```python
from build123d import *

# Parameters (mm, degrees)
SKETCH1_R           = 41.275
SKETCH1_R_2         = 6.5024
SKETCH1_R_3         = 7.62
BOSS_EXTRUDE1_DEPTH = 9.525
SKETCH2_R           = 38.0365
SKETCH2_R_2         = 33.02
BOSS_EXTRUDE2_DEPTH = 63.5
SKETCH3_R           = 12.7
SKETCH3_R_2         = 6.5024
BOSS_EXTRUDE3_DEPTH = 15.875
CHAMFER1_SIZE       = 6.35
CHAMFER1_SIZE2      = 2.54
SKETCH4_R           = 12.7
SKETCH4_R_2         = 6.5024
BOSS_EXTRUDE4_DEPTH = 6.35
FILLET1_R           = 2.54


with BuildPart() as part:
    # Sketch1 → Boss-Extrude1 (new body)
    with BuildSketch(Plane(origin=(0, 0, 0), x_dir=(1, 0, 0), z_dir=(0, 1, 0))):
        Circle(SKETCH1_R)
        Circle(SKETCH1_R_2, mode=Mode.SUBTRACT)
        with Locations((0, 22.86)):
            Circle(SKETCH1_R_3, mode=Mode.SUBTRACT)
        with Locations((21.741151963, 7.064128491)):
            Circle(SKETCH1_R_3, mode=Mode.SUBTRACT)
        with Locations((13.436770867, -18.494128491)):
            Circle(SKETCH1_R_3, mode=Mode.SUBTRACT)
        with Locations((-13.436770867, -18.494128491)):
            Circle(SKETCH1_R_3, mode=Mode.SUBTRACT)
        with Locations((-21.741151963, 7.064128491)):
            Circle(SKETCH1_R_3, mode=Mode.SUBTRACT)
    extrude(amount=BOSS_EXTRUDE1_DEPTH)

    # Sketch2 → Boss-Extrude2 (add)
    with BuildSketch(Plane(origin=(0, 9.525, 0), x_dir=(1, 0, 0), z_dir=(0, 1, 0))):
        Circle(SKETCH2_R)
        Circle(SKETCH2_R_2, mode=Mode.SUBTRACT)
    extrude(amount=BOSS_EXTRUDE2_DEPTH)

    # Sketch3 → Boss-Extrude3 (add)
    with BuildSketch(Plane(origin=(0, 9.525, 0), x_dir=(1, 0, 0), z_dir=(0, 1, 0))):
        Circle(SKETCH3_R)
        Circle(SKETCH3_R_2, mode=Mode.SUBTRACT)
    extrude(amount=BOSS_EXTRUDE3_DEPTH)

    # Chamfer1
    chamfer1_edges = [part.edges().sort_by_distance(p)[0] for p in [
        (-38.0365, 73.025, 0),
    ]]
    chamfer1_side = [part.faces().sort_by_distance(p)[0] for p in [
        (-38.0365, 41.275, 0),
    ]]
    chamfer(chamfer1_edges, length=CHAMFER1_SIZE, length2=CHAMFER1_SIZE2, reference=chamfer1_side[0])

    # Sketch4 → Boss-Extrude4 (add)
    with BuildSketch(Plane(origin=(0, 25.4, 0), x_dir=(1, 0, 0), z_dir=(0, 1, 0))):
        Circle(SKETCH4_R)
        Circle(SKETCH4_R_2, mode=Mode.SUBTRACT)
    extrude(amount=BOSS_EXTRUDE4_DEPTH)

    # Fillet1
    fillet1_edges = [part.edges().sort_by_distance(p)[0] for p in [
        (-12.7, 31.75, 0),
    ]]
    fillet(fillet1_edges, radius=FILLET1_R)


solid = part.part
```
Geometry check sheet. Reference: the model listing, model coordinates, mm. A direction names the side the tool comes from. Coordinates: 2 decimals unless noted, no trailing zeros. Order: outer loops, then holes, each group sorted by start corner. A loop starts at its lowest first (then second) coordinate and runs counter-clockwise, first axis right, second up. Notation, with made-up numbers: M 43,-6 L 67,-6 A7 cw 67,6 Z; hole C 47,65.5 d6. An arc over 180 degrees is marked long. Answer as a JSON object with one key per item and string values.
Q1. Tool access check on faces 4 (the flat face through (0, 9.525, 14)), 5 (the cylindrical face through (-14.47, 4.7, -9.35)). Record the directions out of +Z, -Z, +X, -X, +Y, -Y that give a thin tool (end or side, any length) a straight path to the whole face; none if there is none.
Results are:
{"face 4": "+Y", "face 5": "+Y, -Y"}
Q2. Depth check by flat-ended pin: pin 1 Ø20 at (x, z) = (-21.74, -7.06) entering from -Y; pin 2 Ø12 at (x, z) = (0, -22.86) entering from -Y; pin 3 Ø12 at (x, y) = (11.5, 23.5) entering from -Z; pin 4 Ø10 at (x, y) = (-27.5, 16) entering from -Z. Enter the tip coordinate at first touch or a pass-through.
Results are:
{"pin 1": "stops at y = 0", "pin 2": "passes through", "pin 3": "stops at z = -37.64", "pin 4": "stops at z = -30.67"}
Q3. Cross-section at A-A on x = 0. Give the number of separate pieces and of enclosed holes in the cut face, and give its area (3 significant figures).
Results are:
{"separate pieces": "3", "enclosed holes": "0", "area": "1,410 mm²"}
Q4. Release check for a two-part mould opening along X. For faces 1 (the conical face through (33.975, 72.717, -10.699)), 2 (the flat face through (36.5, 9.525, 12)), 3 (the cylindrical face through (-0.846, 15.653, -6.447)) record: released by +X, released by -X, zero draft, split by the parting line, or undercut.
Results are:
{"face 1": "split by the parting line", "face 2": "zero draft", "face 3": "undercut"}
Q5. Scan lines: line 1 (Z direction, x = 0, y = 7.5) (3 decimals); line 2 (X direction, y = 26, z = -5); line 3 (Z direction, x = 1, y = 52.5). Record each from-to range of solid material in increasing order.
Results are:
{"line 1": "z = -41.275 to -30.48, -15.24 to -6.502, 6.502 to 41.275", "line 2": "x = -37.71 to -32.64, -11.67 to -4.16, 4.16 to 11.67, 32.64 to 37.71", "line 3": "z = -38.02 to -33, 33 to 38.02"}
Q6. Cross-section at C-C on y = 45. Record the cut outline in (x, z).
Results are:
{"outline": "C 0,0 d76.07; hole C 0,0 d66.04"}
Q7. Cross-section at B-B on y = 13. Record the cut outline in (x, z).
Results are:
{"outline": "C 0,0 d76.07; C 0,0 d25.4; hole C 0,0 d66.04; hole C 0,0 d13"}
